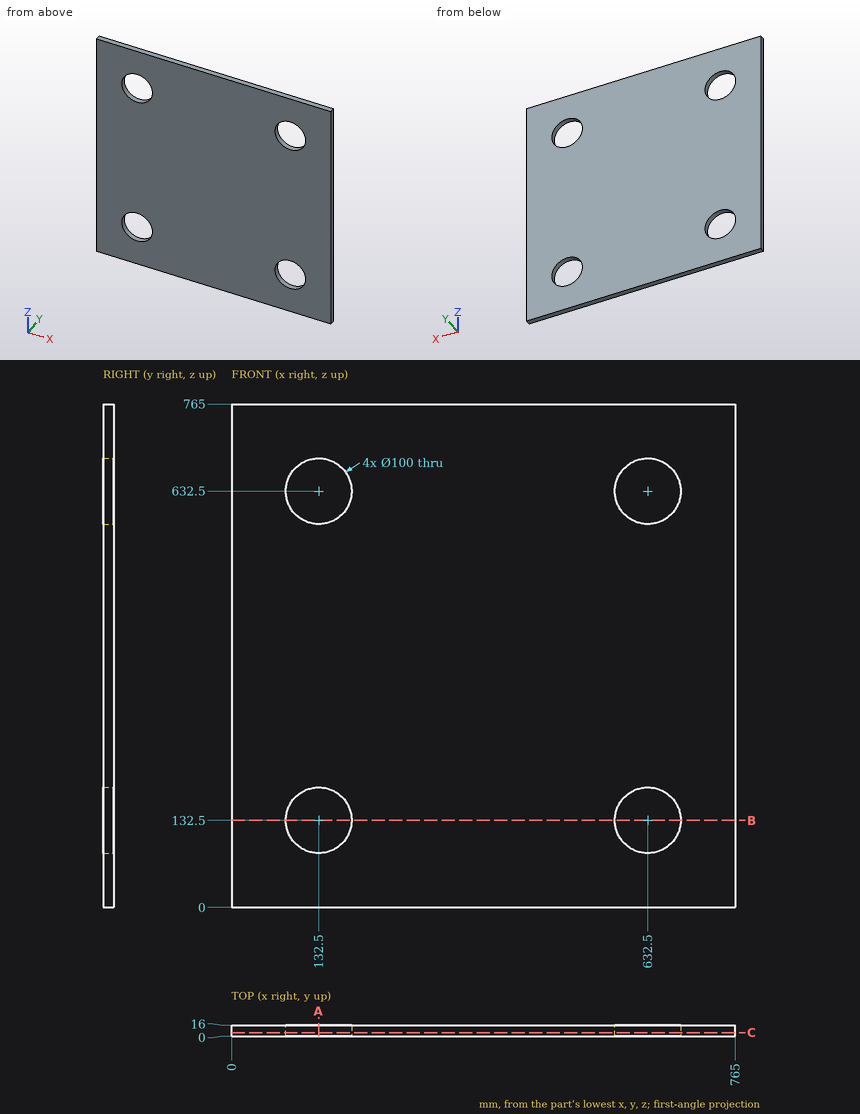
Print and shaded views of the part. All mm, measured from the part's lowest x, y and z. Coordinates: 2 decimals unless noted, no trailing zeros. Write each loop counter-clockwise with the first axis right and the second up, starting at its lowest first coordinate (ties: lowest second). Pieces come first, ordered by that corner, then holes. Notation, with made-up numbers: (9, -37) - (25, -37) arc R24 cw to (25, -15) - close; hole circle Ø3 at (-10.5, 30.25). An arc over 180 degrees is marked (long way). One line per question, with ' | ' between items. Start each with the question number.
Q1. Cut at A-A, the plane x = 132.5. List the corners of the cut face in (y, z).
Q2. Drill centre lines: line 1 (Z direction, x = 132.5, y = 8.75); line 2 (Z direction, x = 669, y = 4). Where is each one in solid material? Low to high. Write a range as [from, to].
Q3. Cut at B-B, the plane z = 132.5. List the corners of the cut face in (x, y).
Q4. Pin check, flat tip, straight feed: pin 1 (5 mm diameter, centred on x = 289.5, z = 394.5, fed in from -Y). Stop position of the tip, or through.
Q5. Cut at C-C, the plane y = 5. List the corners of the cut face in (x, z).
Answer below:
1) outline: (0, 0) - (16, 0) - (16, 82.5) - (0, 82.5) - close; (0, 182.5) - (16, 182.5) - (16, 582.5) - (0, 582.5) - close; (0, 682.5) - (16, 682.5) - (16, 765) - (0, 765) - close
2) line 1: [0, 82.5], [182.5, 582.5], [682.5, 765] | line 2: [0, 98.33], [166.67, 598.33], [666.67, 765]
3) outline: (0, 0) - (82.5, 0) - (82.5, 16) - (0, 16) - close; (182.5, 0) - (582.5, 0) - (582.5, 16) - (182.5, 16) - close; (682.5, 0) - (765, 0) - (765, 16) - (682.5, 16) - close
4) pin 1: y = 0
5) outline: (0, 0) - (765, 0) - (765, 765) - (0, 765) - close; hole circle Ø100 at (132.5, 132.5); hole circle Ø100 at (132.5, 632.5); hole circle Ø100 at (632.5, 132.5); hole circle Ø100 at (632.5, 632.5)
